The model under review builds one solid part; all positions refer to its coordinate system, in mm. Face numbers are marked on the shaded views. A direction names the side the tool comes from. Coordinates: 2 decimals unless noted, no trailing zeros. Loops run counter-clockwise (first coordinate to the right, second up) from the corner with the lowest first, then second, coordinate; pieces in that order, holes last. Notation, with made-up numbers: (26, 68) -> (84, 68) arc R24 ccw to (84, 95) -> close; hole circle Ø5 at (40, 84). An arc over 180 degrees is marked (long way). One line per question, with ' | ' between items. Start each with the question number.
from build123d import *

# Parameters (mm, degrees)
SKETCH_1_W          = 30.8
SKETCH_1_H          = 42
EXTRUDE_1_DEPTH     = 5
SKETCH_2_W          = 30.8
SKETCH_2_H          = 3
EXTRUDE_2_DEPTH     = 8
SKETCH_3_W          = 5
SKETCH_3_H          = 19
EXTRUDE_3_DEPTH     = 8
EXTRUDE_4_DEPTH     = 30.8
CUT_EXTRUDE_1_REACH = 6
SKETCH_5_R          = 1.5
SKETCH_6_W          = 1.45
SKETCH_6_H          = 1
EXTRUDE_5_DEPTH     = 30.8


with BuildPart() as part:
    # 草图1 → 凸台-拉伸1 (new body)
    with BuildSketch(Plane.XY):
        with Locations((15.4, 21)):
            Rectangle(SKETCH_1_W, SKETCH_1_H)
    extrude(amount=EXTRUDE_1_DEPTH)

    # 草图2 → 凸台-拉伸2 (add)
    with BuildSketch(Plane.XY.offset(5)):
        with Locations((15.4, 40.5)):
            Rectangle(SKETCH_2_W, SKETCH_2_H)
        with Locations((15.4, 20.5)):
            Rectangle(SKETCH_2_W, SKETCH_2_H)
    extrude(amount=EXTRUDE_2_DEPTH)

    # 草图3 → 凸台-拉伸3 (add)
    with BuildSketch(Plane.XY.offset(5)):
        with Locations((15.4, 9.5)):
            Rectangle(SKETCH_3_W, SKETCH_3_H)
    extrude(amount=EXTRUDE_3_DEPTH)

    # 草图4 → 凸台-拉伸4 (add)
    with BuildSketch(Plane(origin=(30.8, 0, 0), x_dir=(0, 0, -1), z_dir=(1, 0, 0))):
        Polygon((-5, 0), (-5, -8), (-13, -8), (-13, -12), (0, -12), (0, 0), align=None)
    extrude(amount=-EXTRUDE_4_DEPTH)

    # 草图5 → 切除-拉伸1 (cut, up to next)
    with BuildSketch(Plane(origin=(0, -8, 0), x_dir=(1, 0, 0), z_dir=(0, 1, 0)), mode=Mode.PRIVATE) as cut_extrude_1_sk1:
        with Locations((5, -9)):
            Circle(SKETCH_5_R)
    cut_extrude_1_tool1 = extrude(cut_extrude_1_sk1.sketch, amount=-CUT_EXTRUDE_1_REACH, mode=Mode.PRIVATE) & part.part
    add(cut_extrude_1_tool1.solids().sort_by_distance((5, -8, 9))[0], mode=Mode.SUBTRACT)
    # 草图5 → 切除-拉伸1 (cut, up to next)
    with BuildSketch(Plane(origin=(0, -8, 0), x_dir=(1, 0, 0), z_dir=(0, 1, 0)), mode=Mode.PRIVATE) as cut_extrude_1_sk2:
        with Locations((25.8, -9)):
            Circle(SKETCH_5_R)
    cut_extrude_1_tool2 = extrude(cut_extrude_1_sk2.sketch, amount=-CUT_EXTRUDE_1_REACH, mode=Mode.PRIVATE) & part.part
    add(cut_extrude_1_tool2.solids().sort_by_distance((25.8, -8, 9))[0], mode=Mode.SUBTRACT)

    # 草图6 → 凸台-拉伸5 (add, through all)
    with BuildSketch(Plane(origin=(30.8, 0, 0), x_dir=(0, 0, -1), z_dir=(1, 0, 0))):
        with Locations((-12.275, 38.5)):
            Rectangle(SKETCH_6_W, SKETCH_6_H)
        with Locations((-12.275, 22.5)):
            Rectangle(SKETCH_6_W, SKETCH_6_H)
    extrude(amount=-EXTRUDE_5_DEPTH)


solid = part.part
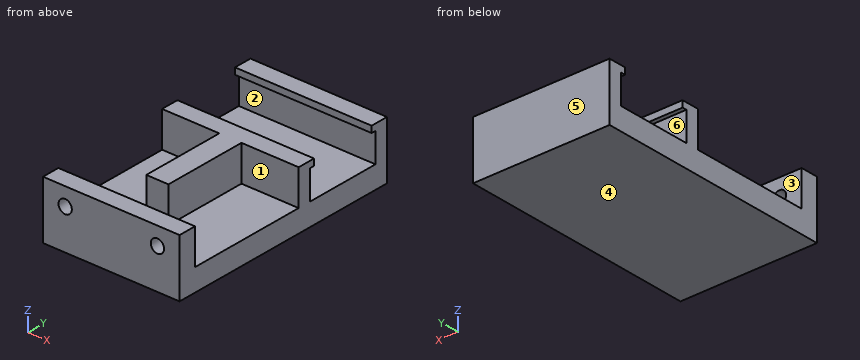
1) Mouldability with a two-part tool opening along Y and no side actions: class the marked faces 4, 5 and 6 as +Y half, -Y half, draft (parallel to the pull), parting line (faces both ways), or undercut.
2) Consider section C-C, the plane y = 8.5. Write out the cut boundary in (x, z), plus the area to 3 significant figures.
3) Consider section B-B, the plane z = 9. Write out the cut boundary in (x, y).
4) Consider section D-D, the plane x = 2. Write out the cut boundary in (y, z), plus the area to 3 significant figures.
5) Insertion check: pin 1 Ø8.5 at (x, y) = (16, 31) entering from +Z; pin 2 Ø6.5 at (y, z) = (8, 8.5) entering from +X; pin 3 Ø6.5 at (y, z) = (10.5, 8.5) entering from -X. Each pin has a flat end and moves straight along its axis. Give the tip position at first contact, or say it passes through.
6) Consider section A-A, the plane x = 25.8. Write out the cut boundary in (y, z).
7) Machinability: for the marked faces 1, 2 and 3, which of the approach directions +Z, -Z, +X, -X, +Y, -Y give a long, thin tool a straight path to every point of the face, cutting with its end or side? Answer none if there is none.
8) Wall thickness on L1, parallel to Y at x = 7, z = 12; L2, parallel to Y at x = 13.5, z = 10; L3, parallel to X at y = -8.9, z = 9: over which ranges is each line inside the solid? List them lowest first.
Filled sheet:
1) face 4: draft | face 5: +Y half | face 6: undercut
2) outline: (0, 0) -> (30.8, 0) -> (30.8, 5) -> (17.9, 5) -> (17.9, 13) -> (12.9, 13) -> (12.9, 5) -> (0, 5) -> close | area: 194 mm^2
3) outline: (0, -12) -> (3.5, -12) -> (3.5, -8) -> (0, -8) -> close; (0, 19) -> (12.9, 19) -> (12.9, 0) -> (17.9, 0) -> (17.9, 19) -> (30.8, 19) -> (30.8, 22) -> (0, 22) -> close; (0, 39) -> (30.8, 39) -> (30.8, 42) -> (0, 42) -> close; (6.5, -12) -> (24.3, -12) -> (24.3, -8) -> (6.5, -8) -> close; (27.3, -12) -> (30.8, -12) -> (30.8, -8) -> (27.3, -8) -> close
4) outline: (-12, 0) -> (42, 0) -> (42, 13) -> (38, 13) -> (38, 11.55) -> (39, 11.55) -> (39, 5) -> (22, 5) -> (22, 11.55) -> (23, 11.55) -> (23, 13) -> (19, 13) -> (19, 5) -> (-8, 5) -> (-8, 13) -> (-12, 13) -> close | area: 353 mm^2
5) pin 1: z = 5 | pin 2: x = 17.9 | pin 3: x = 12.9
6) outline: (-12, 0) -> (42, 0) -> (42, 13) -> (38, 13) -> (38, 11.55) -> (39, 11.55) -> (39, 5) -> (22, 5) -> (22, 11.55) -> (23, 11.55) -> (23, 13) -> (19, 13) -> (19, 5) -> (-8, 5) -> (-8, 7.5) -> (-12, 7.5) -> close; (-12, 10.5) -> (-8, 10.5) -> (-8, 13) -> (-12, 13) -> close
7) face 1: +Z, +X | face 2: +X, -X | face 3: +Z, +X, -X
8) L1: -12 to -8, 19 to 23, 38 to 42 | L2: -12 to -8, 0 to 22, 39 to 42 | L3: 0 to 3.5, 6.5 to 24.3, 27.3 to 30.8
